Work out the finished part from the listing and answer in its coordinate system (mm). A direction names the side the tool comes from. Give positions to 0.01 mm unless a question says otherwise; leave off trailing zeros. Order: outer loops, then holes, each group sorted by start corner. A loop starts at its lowest first (then second) coordinate and runs counter-clockwise, first axis right, second up. Notation, with made-up numbers: M 78.5,-23 L 128.5,-23 A16 cw 128.5,1 Z; hole C 1,47 d11. An arc over 180 degrees is marked long. One line per item, written item: value.
Autodesk Inventor part; units mm, degrees
ref_plane "YZ Plane" through (0, 0, 0) normal (1, 0, 0) x (0, 1, 0)
ref_plane "XZ Plane" through (0, 0, 0) normal (0, 1, 0) x (-1, 0, 0)
ref_plane "XY Plane" through (0, 0, 0) normal (0, 0, 1) x (1, 0, 0)
sketch "Sketch1" plane through (0, 0, 0) normal (0, 0, 1) x (1, 0, 0)
  circle A0 centre (0, 0) radius 1.5
  dimension "d0" = 3
extrude "Extrusion1" add sketch "Sketch1" along normal blind 30
ref_plane "Work Plane1" through (0, 0, 23) normal (0, 0, 1) x (1, 0, 0)
ref_plane "Work Plane2" through (0, 0, 7) normal (0, 0, -1) x (-1, 0, 0)
sketch "Sketch2" plane through (0, 0, 23) normal (0, 0, 1) x (1, 0, 0)
  circle A0 centre (0, 0) radius 1.5
  line L0 (1, 0) -> (-1, 0)
  line L1 (-1, 0) -> (-1, 27.5)
  line L2 (-1, 27.5) -> (1, 27.5)
  line L3 (1, 27.5) -> (1, 0)
  dimension "d7" = 27.5
  dimension "d13" = 1
extrude "Extrusion2" add sketch "Sketch2" against normal up to surface (16 mm away) contours L3 L0 L1 A0 | A0 L1 L2 L3 picked at (0, 0.5)
sketch "Sketch3" plane through (1, 1.118, 23) normal (1, 0, 0) x (0, 0, -1)
  line L0 (16, 0) -> (16, 26.382)
  line L1 (0, 26.382) -> (16, 26.382)
  line L2 (0, 26.382) -> (0, 0)
  line L3 (16, 0) -> (0, 0)
  line L4 (0, 26.382) -> (-7, 26.382)
  line L5 (-7, 26.382) -> (-7, 5.882)
  line L6 (-7, 5.882) -> (0, 5.882)
  line L7 (0, 5.882) -> (0, 26.382)
  line L8 (16, 0) -> (16, 26.382)
  line L9 (16, 26.382) -> (23, 26.382)
  line L10 (23, 26.382) -> (23, 5.882)
  line L11 (23, 5.882) -> (16, 5.882)
  line L12 (16, 5.882) -> (16, 26.382)
  line L13 (23, -2.618) -> (23, 0.382)
  line L14 (-7, 0.382) -> (-7, -2.618)
  line L15 (0, 0) -> (16, 0)
  line L16 (16, 0) -> (16, 0)
  line L17 (16, 0) -> (0, 0)
  line L18 (0, 0) -> (0, 0)
  point P0 (23, -1.118)
  point P1 (19.5, 5.882)
  point P2 (-3.5, 5.882)
  point P3 (23, -1.118)
  point P4 (23, 16.132)
  point P5 (-7, 16.132)
  point P6 (-7, -1.118)
  dimension "d10" = 5.5
extrude "Extrusion3" add sketch "Sketch3" against normal up to surface (2 mm away) contours L0 L9 L10 L11 | L6 L5 L4 L2
sketch "Sketch5" plane through (-1, 1.118, 7) normal (-1, 0, 0) x (0, 0, 1)
  line L0 (16, 0) -> (0, 0)
  line L1 (16, 0) -> (16, 5.882)
  line L2 (23, 5.882) -> (16, 5.882)
  line L3 (23, 26.382) -> (23, 5.882)
  line L4 (23, 26.382) -> (-7, 26.382)
  line L5 (-7, 5.882) -> (-7, 26.382)
  line L6 (0, 5.882) -> (-7, 5.882)
  line L7 (0, 5.882) -> (0, 0)
  line L8 (23, 5.882) -> (16, 5.882)
  line L9 (23, 26.382) -> (-7, 26.382)
  line L10 (23, 5.882) -> (20.5, 5.882)
  line L11 (20.5, 5.882) -> (20.5, 26.382)
  line L12 (20.5, 26.382) -> (23, 26.382)
  line L13 (23, 26.382) -> (23, 5.882)
  line L14 (0, 5.882) -> (-7, 5.882)
  line L15 (-7, 26.382) -> (-2.6, 26.382)
  line L16 (-2.6, 26.382) -> (-2.6, 5.882)
  line L17 (-2.6, 5.882) -> (-7, 5.882)
  line L18 (-7, 5.882) -> (-7, 26.382)
  point P0 (-7, -1.118)
  dimension "d16" = 2.5
  dimension "d17" = 4.4
extrude "Extrusion5" add sketch "Sketch5" along normal blind 1.26 contours L11 L4 L3 L2 | L6 L5 L4 L16
properties part number "gpsDoor"
(1) Find the intervals of material crossed by probe 1 along Z at (x, y) = (-1.25, 8); probe 2 along X at (y, z) = (15.5, 24); probe 3 along X at (y, z) = (16, 28.25), in increasing order. Write a range as from..to.
Findings:
probe 1: z = 0..4.4, 27.5..30
probe 2: x = -1..1
probe 3: x = -2.26..1
(2) Section B-B, the plane z = 23.75 is taken. Give the vertices of the cut face in (x, y), then the cut area to 3 significant figures.
Findings:
outline: C 0,0 d3; M -1,7 L 1,7 L 1,27.5 L -1,27.5 Z
area: 48.1 mm^2
(3) Section A-A, the plane x = 0 is taken. Give the vertices of the cut face in (y, z), then the cut area to 3 significant figures.
Findings:
outline: M -1.5,0 L 1.5,0 L 1.5,7 L 7,7 L 7,0 L 27.5,0 L 27.5,30 L 7,30 L 7,23 L 1.5,23 L 1.5,30 L -1.5,30 Z
area: 793 mm^2
(4) Section D-D, the plane z = 17.75 is taken. Give the vertices of the cut face in (x, y), then the cut area to 3 significant figures.
Findings:
outline: M -1,1.12 A1.5 ccw long 1,1.12 L 1,27.5 L -1,27.5 Z
area: 59.3 mm^2
(5) Given P1, Ø1.6, axis at x = -1.5, z = 28, coming from the -Y side; P2, Ø13, axis at y = 13.5, z = 16.5, coming from the +X side; P3, Ø7, axis at y = 16.5, z = 15, coming from the -X side, each flat-ended and moving along its own axis, determine where each tip first touches the part or whether it passes through.
Findings:
P1: stops at y = -1.33
P2: stops at x = 1
P3: stops at x = -1
(6) Determine the mould class of faces 5 (the flat face through (0, 4, 7)), 6 (the flat face through (-1, 7, 3)), 7 (the flat face through (0, 27.5, 15)), 8 (the flat face through (-2.26, 17, 29)) for opening direction Y: pulls with the +Y half, pulls with the -Y half, needs draft (parallel to the pull), parting line crosses it, or undercut.
Findings:
face 5: undercut
face 6: undercut
face 7: pulls with the +Y half
face 8: needs draft
(7) Section C-C, the plane y = 22.5 is taken. Give the vertices of the cut face in (x, z), then the cut area to 3 significant figures.
Findings:
outline: M -2.26,0 L 1,0 L 1,30 L -2.26,30 L -2.26,27.5 L -1,27.5 L -1,4.4 L -2.26,4.4 Z
area: 68.7 mm^2
(8) Which of the six approach directions +Z, -Z, +X, -X, +Y, -Y give full straight-line access (tool end or side, diameter ignored) to faces 1 (the flat face through (0, 7, 27)), 2 (the flat face through (1, 14, 15)), 3 (the flat face through (-1, 14, 16)), 4 (the flat face through (0, 0, 0))?
Findings:
face 1: +Z, +X, -X
face 2: +Z, -Z, +X, +Y
face 3: -X, +Y
face 4: -Z, +X, -X, +Y, -Y
